Could you check a few things on this drawing? It's one solid part, dimensions in mm from its lowest x, y, z. A direction names the side the tool comes from. Round coordinates to 2 decimals unless told otherwise and drop trailing zeros. Write each loop counter-clockwise with the first axis right and the second up, starting at its lowest first coordinate (ties: lowest second). Pieces come first, ordered by that corner, then holes. Notation, with made-up numbers: (-16.75, 45) - (20.25, 45) arc R23 ccw to (20.25, 77) - close; hole circle Ø9 at (72, -23.75). An arc over 180 degrees is marked (long way). Put each result on its own line as item: value.
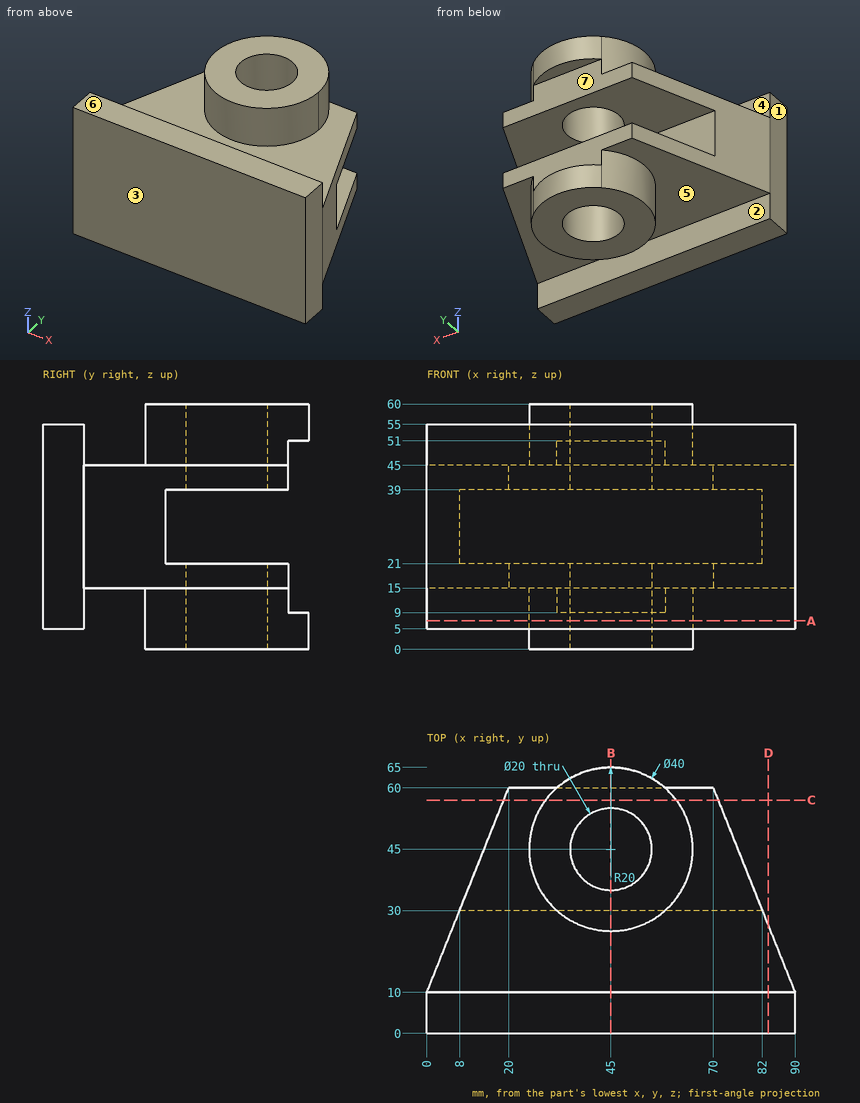
(1) If we mould it in two halves opening along Y, with no side actions, what happens to the marked faces 1, 2 and 3? For each: pulls with the +Y half, pulls with the -Y half, needs draft (parallel to the pull), parting line crosses it, or undercut.
Values found:
face 1: needs draft
face 2: undercut
face 3: pulls with the -Y half
(2) Imagine slicing it at D-D, the plane x = 83.5. List the corners of the cut face in (y, z) for me.
Values found:
outline: (0, 5) - (10, 5) - (10, 15) - (26.25, 15) - (26.25, 45) - (10, 45) - (10, 55) - (0, 55) - close
(3) Imagine slicing it at C-C, the plane y = 57. List the corners of the cut face in (x, z) for me.
Values found:
outline: (18.8, 15) - (29, 15) - (29, 0) - (61, 0) - (61, 15) - (71.2, 15) - (71.2, 21) - (18.8, 21) - close; (18.8, 39) - (71.2, 39) - (71.2, 45) - (61, 45) - (61, 60) - (29, 60) - (29, 45) - (18.8, 45) - close
(4) Imagine slicing it at A-A, the plane z = 7. List the corners of the cut face in (x, y) for me.
Values found:
outline: (0, 0) - (90, 0) - (90, 10) - (0, 10) - close; circle Ø40 at (45, 45); hole circle Ø20 at (45, 45)
(5) For the marked faces 4, 5, 6 and 7, which set-ups out of +Z, -Z, +X, -X, +Y, -Y let a thin tool reach every point of the face, with its end or its side?
Values found:
face 4: +Z, +X, -X
face 5: -Z
face 6: +Z, +X, -X, -Y
face 7: +X, -X, +Y
(6) Please list where these lines run through material, in increasing order: probe 1 along Y at (x, z) = (45, 10); probe 2 along Y at (x, z) = (45, 5.25); probe 3 along Y at (x, z) = (45, 43.5). Write a range as from..to.
Values found:
probe 1: y = 0..10, 25..35, 55..60
probe 2: y = 0..10, 25..35, 55..65
probe 3: y = 0..35, 55..60
(7) I'm going to push flat-ended pins straight in: pin 1 (10 mm diameter, centred on y = 30, z = 44, fed in from +X); pin 2 (23 mm diameter, centred on x = 45, y = 45, fed in from +Z); pin 3 (9 mm diameter, centred on x = 38.5, z = 28.5, fed in from +Y); pin 4 (9.5 mm diameter, centred on x = 46.5, z = 46.5, fed in from +Y). Where does each tip first touch, or does it pass through?
Values found:
pin 1: stops at x = 84
pin 2: stops at z = 60
pin 3: stops at y = 30
pin 4: stops at y = 65
(8) Imagine slicing it at B-B, the plane x = 45. List the corners of the cut face in (y, z) for me, then the cut area to 3 significant figures.
Values found:
outline: (0, 5) - (10, 5) - (10, 15) - (25, 15) - (25, 0) - (35, 0) - (35, 21) - (30, 21) - (30, 39) - (35, 39) - (35, 60) - (25, 60) - (25, 45) - (10, 45) - (10, 55) - (0, 55) - close; (55, 0) - (65, 0) - (65, 9) - (60, 9) - (60, 21) - (55, 21) - close; (55, 39) - (60, 39) - (60, 51) - (65, 51) - (65, 60) - (55, 60) - close
area: 1,760 mm^2
